Geometry check sheet. Reference: the model listing, model coordinates, mm. Coordinates: 2 decimals unless noted, no trailing zeros. Write each loop counter-clockwise with the first axis right and the second up, starting at its lowest first coordinate (ties: lowest second). Pieces come first, ordered by that corner, then holes.
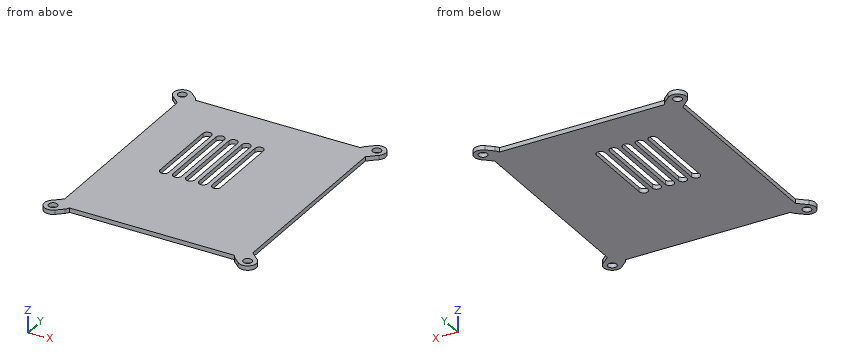
Autodesk Inventor part; units mm, degrees
ref_plane "YZ Plane" through (0, 0, 0) normal (1, 0, 0) x (0, 1, 0)
ref_plane "XZ Plane" through (0, 0, 0) normal (0, 1, 0) x (-1, 0, 0)
ref_plane "XY Plane" through (0, 0, 0) normal (0, 0, 1) x (1, 0, 0)
sketch "Sketch1" plane through (0, 0, 0) normal (0, 0, 1) x (1, 0, 0)
  circle A0 centre (44.8094, -51.3621) radius 1.985
  circle A1 centre (-44.8094, -51.3621) radius 1.985
  circle A2 centre (-44.8094, 51.3621) radius 1.985
  circle A3 centre (44.8094, 51.3621) radius 1.985
  line L0 (38.0119, 50.05) -> (-38.0119, 50.05)
  arc A4 (-38.0119, 50.05) -> (-39.1663, 51.7567) centre (-41.7906, 48.7379) ccw
  line L1 (-42.1852, 54.381) -> (-39.1663, 51.7567)
  arc A5 (-42.1852, 54.381) -> (-47.4337, 48.3433) centre (-44.8094, 51.3621) ccw
  line L2 (-43.3, 44.7499) -> (-47.4337, 48.3433)
  line L3 (-43.3, 44.7499) -> (-43.3, -44.7499)
  line L4 (-47.4337, -48.3433) -> (-43.3, -44.7499)
  arc A6 (-47.4337, -48.3433) -> (-42.1852, -54.381) centre (-44.8094, -51.3621) ccw
  line L5 (-39.1663, -51.7567) -> (-42.1852, -54.381)
  arc A7 (-39.1663, -51.7567) -> (-38.0119, -50.05) centre (-41.7906, -48.7379) ccw
  line L6 (-38.0119, -50.05) -> (38.0119, -50.05)
  arc A8 (38.0119, -50.05) -> (39.1663, -51.7567) centre (41.7906, -48.7379) ccw
  line L7 (42.1852, -54.381) -> (39.1663, -51.7567)
  arc A9 (42.1852, -54.381) -> (47.4337, -48.3433) centre (44.8094, -51.3621) ccw
  line L8 (43.3, -44.7499) -> (47.4337, -48.3433)
  line L9 (43.3, -44.7499) -> (43.3, 44.7499)
  line L10 (47.4337, 48.3433) -> (43.3, 44.7499)
  arc A10 (47.4337, 48.3433) -> (42.1852, 54.381) centre (44.8094, 51.3621) ccw
  line L11 (39.1663, 51.7567) -> (42.1852, 54.381)
  arc A11 (39.1663, 51.7567) -> (38.0119, 50.05) centre (41.7906, 48.7379) ccw
  line L12 (-40.1, -44.85) -> (-40.1, 44.85)
  arc A12 (-38.1, 46.85) -> (-40.1, 44.85) centre (-38.1, 44.85) ccw
  line L13 (-38.1, 46.85) -> (38.1, 46.85)
  arc A13 (40.1, 44.85) -> (38.1, 46.85) centre (38.1, 44.85) ccw
  line L14 (40.1, 44.85) -> (40.1, -44.85)
  arc A14 (38.1, -46.85) -> (40.1, -44.85) centre (38.1, -44.85) ccw
  line L15 (38.1, -46.85) -> (-38.1, -46.85)
  arc A15 (-40.1, -44.85) -> (-38.1, -46.85) centre (-38.1, -44.85) ccw
  point P0 (0, 0)
extrude "Extrusion1" add sketch "Sketch1" along normal blind 2 contours A11 L11 A10 L10 L9 L8 A9 L7 A8 L6 A7 L5 A6 L4 L3 L2 A5 L1 A4 L0 | L12 A12 L13 A13 L14 A14 L15 A15
sketch "Sketch3" plane through (0, 0, 2) normal (0, 0, 1) x (1, 0, 0)
  line L0 (-15.2986, 18.4674) -> (-1.1867, 18.4674)
  line L1 (-1.1867, 18.4674) -> (-1.1867, 4.4942)
  line L2 (-1.1867, 4.4942) -> (-15.2986, 4.4942)
  line L3 (-15.2986, 4.4942) -> (-15.2986, 18.4674)
  line L4 (-8.1427, -5.5192) -> (-8.1427, 28.4808) construction
  line L5 (-6.1427, -5.5192) -> (-6.1427, 28.4808)
  line L6 (-10.1427, 28.4808) -> (-10.1427, -5.5192)
  arc A0 (-10.1427, -5.5192) -> (-6.1427, -5.5192) centre (-8.1427, -5.5192) ccw
  arc A1 (-6.1427, 28.4808) -> (-10.1427, 28.4808) centre (-8.1427, 28.4808) ccw
  arc A2 (-0.1427, 28.4808) -> (-4.1427, 28.4808) centre (-2.1427, 28.4808) ccw
  line L7 (-0.1427, -5.5192) -> (-0.1427, 28.4808)
  line L8 (-4.1427, 28.4808) -> (-4.1427, -5.5192)
  arc A3 (-4.1427, -5.5192) -> (-0.1427, -5.5192) centre (-2.1427, -5.5192) ccw
  line L9 (5.8573, -5.5192) -> (5.8573, 28.4808)
  arc A4 (5.8573, 28.4808) -> (1.8573, 28.4808) centre (3.8573, 28.4808) ccw
  line L10 (1.8573, 28.4808) -> (1.8573, -5.5192)
  arc A5 (1.8573, -5.5192) -> (5.8573, -5.5192) centre (3.8573, -5.5192) ccw
  line L11 (-16.1427, 28.4808) -> (-16.1427, -5.5192)
  arc A6 (-12.1427, 28.4808) -> (-16.1427, 28.4808) centre (-14.1427, 28.4808) ccw
  line L12 (-12.1427, -5.5192) -> (-12.1427, 28.4808)
  arc A7 (-16.1427, -5.5192) -> (-12.1427, -5.5192) centre (-14.1427, -5.5192) ccw
  line L13 (-22.1427, 28.4808) -> (-22.1427, -5.5192)
  arc A8 (-18.1427, 28.4808) -> (-22.1427, 28.4808) centre (-20.1427, 28.4808) ccw
  line L14 (-18.1427, -5.5192) -> (-18.1427, 28.4808)
  arc A9 (-22.1427, -5.5192) -> (-18.1427, -5.5192) centre (-20.1427, -5.5192) ccw
  point P0 (0, 0)
  point P1 (-8.1427, 11.4808)
  dimension "d8" = 17
  dimension "d9" = 4
  dimension "d12" = 6
  dimension "d19" = 6
  dimension "d26" = 6
extrude "Extrusion3" cut sketch "Sketch3" against normal up to surface (2 mm away) contours L3 L2 L12 A7 L11 A6 L0 | L0 L12 L2 L3 | L6 A1 L5 L0 | L0 L5 L2 L6 | L2 L5 A0 L6 | L8 A2 L7 A3 L2 L1 L0 | L0 L1 L2 L8 | A5 L10 A4 L9 | A8 L14 A9 L13
properties part number "Case Cover Rev D"
1. Sectioned sample at A-A, the plane y = 17.5. Record the boundary of the cut face in (x, z).
Computed values:
outline: (-43.3, 0) - (-22.14, 0) - (-22.14, 2) - (-43.3, 2) - close; (-18.14, 0) - (-16.14, 0) - (-16.14, 2) - (-18.14, 2) - close; (-12.14, 0) - (-10.14, 0) - (-10.14, 2) - (-12.14, 2) - close; (-6.14, 0) - (-4.14, 0) - (-4.14, 2) - (-6.14, 2) - close; (-0.14, 0) - (1.86, 0) - (1.86, 2) - (-0.14, 2) - close; (5.86, 0) - (43.3, 0) - (43.3, 2) - (5.86, 2) - close
2. Sectioned sample at D-D, the plane z = 1. Give the number of separate pieces and of enclosed holes in the cut face, and give its area (3 significant figures).
Computed values:
separate pieces: 1
enclosed holes: 9
area: 8,100 mm2
3. Gauge pin test, flat ends, axial feed: pin 1 Ø1.5 at (x, y) = (-21, 2) entering from -Z; pin 2 Ø1 at (y, z) = (20.5, 0.5) entering from +X; pin 3 Ø1 at (x, z) = (15, 1) entering from +Y; pin 4 Ø1 at (x, z) = (-10, 0) entering from -Y. Record the tip position at first contact, or that the pin passes through.
Computed values:
pin 1: passes through
pin 2: stops at x = 43.3
pin 3: stops at y = 50.05
pin 4: stops at y = -50.05
4. Sectioned sample at B-B, the plane x = 31. Record the boundary of the cut face in (y, z).
Computed values:
outline: (-50.05, 0) - (50.05, 0) - (50.05, 2) - (-50.05, 2) - close
5. Sectioned sample at C-C, the plane y = -12. Record the boundary of the cut face in (x, z), and give its area (3 significant figures).
Computed values:
outline: (-43.3, 0) - (43.3, 0) - (43.3, 2) - (-43.3, 2) - close
area: 173 mm2
6. Thickness scan on line 1 along X through (y, z) = (7, 1.5); line 2 along Y through (x, z) = (11, 1.35); line 3 along X through (y, z) = (-51, 0.3). Record the ranges inside material, lowest first.
Computed values:
line 1: x = -43.3 to -22.14, -18.14 to -16.14, -12.14 to -10.14, -6.14 to -4.14, -0.14 to 1.86, 5.86 to 43.3
line 2: y = -50.05 to 50.05
line 3: x = -48.79 to -46.76, -42.86 to -38.49, 38.49 to 42.86, 46.76 to 48.79
